Autodesk Inventor part; units mm, degrees
ref_plane "YZ Plane" through (0, 0, 0) normal (1, 0, 0) x (0, 1, 0)
ref_plane "XZ Plane" through (0, 0, 0) normal (0, 1, 0) x (-1, 0, 0)
ref_plane "XY Plane" through (0, 0, 0) normal (0, 0, 1) x (1, 0, 0)
sketch "Sketch1" plane through (0, 0, 0) normal (0, 1, 0) x (-1, 0, 0)
  line L0 (0, 0) -> (558.8, 0)
  line L1 (0, 292.1) -> (0, 0)
  arc A0 (6.35, 152.4) -> (292.1, 152.4) centre (149.225, 152.4) ccw
  line L2 (292.1, 152.4) -> (292.1, 241.3)
  line L3 (6.35, 152.4) -> (6.35, 292.1)
  line L4 (0, 292.1) -> (6.35, 292.1)
  line L5 (292.1, 241.3) -> (302.6441, 241.3)
  line L6 (558.8, 0) -> (558.8, 63.5)
  line L7 (558.8, 63.5) -> (302.6441, 241.3)
  point P0 (297.372, 241.3)
  dimension "d0" = 558.8
  dimension "d3" = 285.75
  dimension "d10" = 292.1
  dimension "d14" = 63.5
  dimension "d33" = 241.3
  dimension "d34" = 139.7
  dimension "d37" = 6.35
extrude "Extrusion2" add sketch "Sketch1" along normal blind 3.175
sketch "Sketch2" plane through (-558.8, 0, 0) normal (-1, 0, 0) x (0, 0, 1)
  line L0 (0, 0) -> (63.5, 0)
  line L1 (63.5, 0) -> (63.5, 3.175)
  line L2 (0, 3.175) -> (63.5, 3.175)
  line L3 (0, 0) -> (0, 3.175)
  line L4 (6.35, 0) -> (6.35, 3.175)
  line L5 (19.05, 3.175) -> (19.05, 0)
  line L6 (57.15, 3.175) -> (57.15, 0)
  line L7 (44.45, 3.175) -> (44.45, 0)
  dimension "d15" = 6.35
  dimension "d16" = 12.7
  dimension "d17" = 12.7
  dimension "d18" = 6.35
extrude "Extrusion3" cut sketch "Sketch2" against normal blind 3.175 contours L4 L2 L5 L0 | L7 L2 L6 L0
sketch "Sketch3" plane through (-558.8, 0, 63.5) normal (-0.5702096, 0, 0.8214993) x (0.8214993, 0, 0.5702096)
  line L0 (0, 0) -> (311.8152, 0)
  line L1 (311.8152, 0) -> (311.8152, 3.175)
  line L2 (0, 3.175) -> (311.8152, 3.175)
  line L3 (0, 0) -> (0, 3.175)
  line L4 (6.35, 0) -> (6.35, 3.175)
  line L5 (19.05, 3.175) -> (19.05, 0)
  line L6 (305.4652, 3.175) -> (305.4652, 0)
  line L7 (292.7652, 3.175) -> (292.7652, 0)
  point P0 (422.8455, 0)
  dimension "d21" = 12.7
  dimension "d22" = 6.35
  dimension "d23" = 6.35
  dimension "d24" = 12.7
extrude "Extrusion4" cut sketch "Sketch3" against normal blind 3.175 contours L4 L2 L5 L0 | L7 L2 L6 L0
sketch "Sketch4" plane through (0, 0, 292.1) normal (1, 0, 0) x (0, 0, -1)
  line L0 (0, 0) -> (292.1, 0)
  line L1 (292.1, 0) -> (292.1, 3.175)
  line L2 (0, 3.175) -> (292.1, 3.175)
  line L3 (285.75, 3.175) -> (285.75, 0)
  line L4 (273.05, 3.175) -> (273.05, 0)
  line L5 (6.35, 3.175) -> (6.35, 0)
  line L6 (19.05, 3.175) -> (19.05, 0)
  dimension "d27" = 12.7
  dimension "d28" = 12.7
  dimension "d29" = 6.35
  dimension "d30" = 254
extrude "Extrusion5" cut sketch "Sketch4" against normal blind 3.175 contours L5 L2 L6 L0 | L4 L2 L3 L0
properties part number "Top" material "Polycarbonate, Clear"
Could you check a few things on this model? Use its own coordinates, in mm. Round coordinates to 2 decimals unless told otherwise and drop trailing zeros. Loops run counter-clockwise (first coordinate to the right, second up) from the corner with the lowest first, then second, coordinate; pieces in that order, holes last. Notation, with made-up numbers: M 22,-18 L 33,-18 A24 cw 33,3 Z; hole C 75,-35.75 d8. An arc over 180 degrees is marked long. Write item = value, one per line.
1. Thinking about a two-plate mould opening in X: for faces 1 (the face through (-432.296, 1.565, 151.307)), 2 (the face through (-152.37, 1.57, 9.56)), 3 (the face through (-340, 3.175, 82)), which applies, +X half, -X half, draft (parallel to the pull), parting line (faces both ways), or undercut?
Results below:
face_1 = -X half
face_2 = undercut
face_3 = draft
2. I want a section at C-C, the plane x = -212.5. Write out the boundary of the cut face in (y, z) (3 decimals).
Results below:
outline = M 0,0 L 3.175,0 L 3.175,24.3 L 0,24.3 Z
3. I need wall thicknesses on probe 1 along X at (y, z) = (2.6, 154.5); probe 2 along X at (y, z) = (2.8, 125); probe 3 along Z at (x, y) = (-296.5, 1.8). Which ranges of each line are inside material? Lowest first, please.
Results below:
probe_1 = -427.7 to -292.1, -6.35 to 0
probe_2 = -470.2 to -289.45, -9 to 0
probe_3 = 0 to 241.3
4. Will these pins go through, and if not, where does the flat tip stop? P1, Ø1.6, axis at x = -298.5, y = 2, coming from the +Z side; P2, Ø1.6, axis at y = 1.5, z = 222, coming from the -X side; P3, Ø1, axis at x = -557, y = 2, coming from the +Z side.
Results below:
P1 = 241.3
P2 = -331.6
P3 = 65.1
5. I want a section at A-A, the plane z = 214. Write out the boundary of the cut face in (x, y) (3 decimals), and give its area (3 significant figures).
Results below:
outline = M -341.975,0 L -292.1,0 L -292.1,3.175 L -341.975,3.175 Z; M -6.35,0 L 0,0 L 0,3.175 L -6.35,3.175 Z
area = 179 mm²
6. I want a section at D-D, the plane x = -402.5. Write out the boundary of the cut face in (y, z) (3 decimals), and give its area (3 significant figures).
Results below:
outline = M 0,0 L 3.175,0 L 3.175,171.989 L 0,171.989 Z
area = 546 mm²
